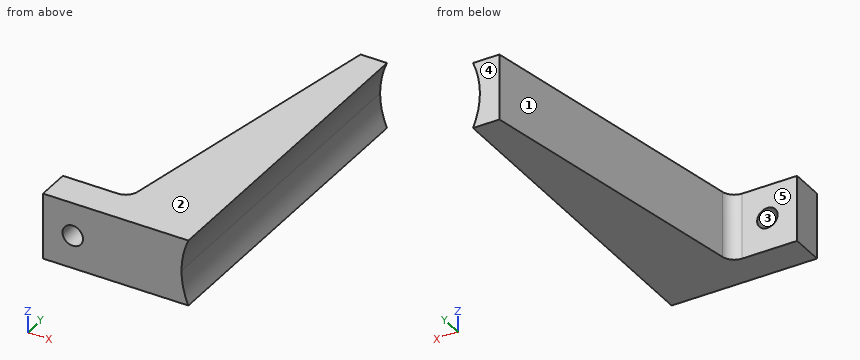
from build123d import *

# Parameters (mm, degrees)
F1_DEPTH = 10
F3_DEPTH = 50.001
F5_D     = 3.1
F6_R     = 2


with BuildPart() as f1:
    # F0 (on Top) → F1 (new body)
    with BuildSketch(Plane.XY):
        Polygon((0, 5), (0, 0), (22, 0), (22, 50), (18, 50), (10, 5), align=None)
    extrude(amount=F1_DEPTH)

    # F2 (on face) → F3 (cut, through all)
    with BuildSketch(Plane(origin=(0, 50, 0), x_dir=(-1, 0, 0), z_dir=(0, 1, 0))):
        with BuildLine():
            Line((-22, 0), (-22, 10))
            ThreePointArc((-22, 10), (-45.956439, 5), (-22, 0))
        make_face()
        with BuildLine():
            ThreePointArc((-22, 0), (-21.22011, 2.446129), (-20.956439, 5))
            ThreePointArc((-20.956439, 5), (-21.22011, 7.553871), (-22, 10))
            Line((-22, 10), (-22, 0))
        make_face()
    extrude(amount=-F3_DEPTH, mode=Mode.SUBTRACT)

    # F5 (through all)
    with Locations(Plane(origin=(0, 5, 0), x_dir=(-1, 0, 0), z_dir=(0, 1, 0))):
        with Locations((-4.5, 5)):
            Hole(F5_D / 2)

    # F6
    f6_edges = [f1.edges().sort_by_distance(p)[0] for p in [
        (10, 5, 5),
    ]]
    fillet(f6_edges, radius=F6_R)


solid = f1.part
Geometry: final body of the model. Coordinates: model frame, mm. Face numbers are marked on the shaded views. A direction names the side the tool comes from. Give positions to 0.01 mm unless a question says otherwise; leave off trailing zeros. Write each loop counter-clockwise with the first axis right and the second up, starting at its lowest first coordinate (ties: lowest second). Pieces come first, ordered by that corner, then holes. Notation, with made-up numbers: (16.25, 29) - (73.25, 29) arc R15 ccw to (73.25, 57) - close; hole circle Ø5 at (17, 67.5). An arc over 180 degrees is marked (long way). Return JSON: item names as keys, results as strings. Group by question number.
1) Set-up query: the marked faces 4 and 5. Return all of +Z, -Z, +X, -X, +Y, -Y with unobstructed straight access to the full face (end or side cutting, diameter ignored); none if empty.
2) Section D-D on x = 6.75. Return the cut outline in (y, z).
3) Section A-A on x = 4.5. Return the cut outline in (y, z), plus the area to 3 significant figures.
4) Line query: line 1 (Z direction, x = 4.5, y = 3.7); line 2 (Y direction, x = 7.75, z = 1.5); line 3 (X direction, y = 5.5, z = 9.75). Output: solid intervals per line, ascending.
5) Mould query, pull axis Z, two halves, no side actions, for the marked faces 1, 2 and 3. Classes: released by +Z, released by -Z, zero draft, split by the parting line, or undercut.
6) Section C-C on z = 2. Return the cut outline in (x, y), plus the area to 3 significant figures.
7) First-contact query: P1, Ø3, axis at y = 31, z = 3, coming from the -X side; P2, Ø1, axis at y = 10, z = 3, coming from the +X side; P3, Ø4, axis at y = 27.5, z = 3.5, coming from the +X side. Flat tips, straight axial feed; report the tip coordinate or a pass-through.
8) Section B-B on y = 32. Return the cut outline in (x, z).
Filled in:
{
 "1": {"face 4": "+Z, -Z, +X, -X, +Y", "face 5": "+Z, -Z, -X, +Y"},
 "2": {"outline": "(0, 0) - (5, 0) - (5, 10) - (0, 10) - close"},
 "3": {"outline": "(0, 0) - (5, 0) - (5, 3.45) - (0, 3.45) - close; (0, 6.55) - (5, 6.55) - (5, 10) - (0, 10) - close", "area": "34.5 mm^2"},
 "4": {"line 1": "z = 0 to 3.45, 6.55 to 10", "line 2": "y = 0 to 5", "line 3": "x = 9.65 to 21.89"},
 "5": {"face 1": "zero draft", "face 2": "released by +Z", "face 3": "undercut"},
 "6": {"outline": "(0, 0) - (21.32, 0) - (21.32, 50) - (18, 50) - (10.29, 6.65) arc R2 cw to (8.32, 5) - (0, 5) - close", "area": "437 mm^2"},
 "7": {"P1": "stops at x = 14.36", "P2": "stops at x = 21.21", "P3": "stops at x = 21.46"},
 "8": {"outline": "(14.8, 0) - (22, 0) arc R12.5 cw to (20.96, 5) arc R12.5 cw to (22, 10) - (14.8, 10) - close"}
}
